Here's how the part is built. I have some questions about the finished solid (model axes, mm). A direction names the side the tool comes from. Give positions to 0.01 mm unless a question says otherwise; leave off trailing zeros. Write each loop counter-clockwise with the first axis right and the second up, starting at its lowest first coordinate (ties: lowest second). Pieces come first, ordered by that corner, then holes. Notation, with made-up numbers: (62, 6.5) - (88, 6.5) arc R18 cw to (88, 30.5) - close; hole circle Ø4 at (22.25, 8.25). An arc over 180 degrees is marked (long way). Use a Markdown table: item, result.
```python
from build123d import *

# Parameters (mm, degrees)
SKETCH1_W           = 20
SKETCH1_H           = 24
BOSS_EXTRUDE1_DEPTH = 3.5
SKETCH2_W           = 16
SKETCH2_H           = 22
CUT_EXTRUDE1_DEPTH  = 0.4
SKETCH3_R           = 1.5
CUT_EXTRUDE2_DEPTH  = 17.007810594
SKETCH4_R           = 2.5
CUT_EXTRUDE3_DEPTH  = 1
SKETCH5_R           = 1
BOSS_EXTRUDE2_DEPTH = 2


with BuildPart() as part:
    # Sketch1 → Boss-Extrude1 (new body)
    with BuildSketch(Plane.XY):
        Rectangle(SKETCH1_W, SKETCH1_H)
    extrude(amount=BOSS_EXTRUDE1_DEPTH)

    # Sketch2 → Cut-Extrude1 (cut)
    with BuildSketch(Plane(origin=(0, 0, 0), x_dir=(-1, 0, 0), z_dir=(0, 0, -1))):
        Rectangle(SKETCH2_W, SKETCH2_H)
    extrude(amount=-CUT_EXTRUDE1_DEPTH, mode=Mode.SUBTRACT)

    # Sketch3 → Cut-Extrude2 (cut, through all)
    with BuildSketch(Plane.XY.offset(3.5)):
        with Locations((0, 3)):
            Circle(SKETCH3_R)
        with Locations((0, 9)):
            Circle(SKETCH3_R)
        with Locations(Location((0, -9, 0), (0, 0, 180))):
            Circle(SKETCH3_R)
        with Locations(Location((0, -3, 0), (0, 0, 180))):
            Circle(SKETCH3_R)
    extrude(amount=-CUT_EXTRUDE2_DEPTH, mode=Mode.SUBTRACT)

    # Sketch4 → Cut-Extrude3 (cut)
    with BuildSketch(Plane.XY.offset(3.5)):
        with Locations((0, 9)):
            Circle(SKETCH4_R)
    cut_extrude3 = extrude(amount=-CUT_EXTRUDE3_DEPTH, mode=Mode.SUBTRACT)

    # Sketch-Pattern1: Cut-Extrude3 at 3 more places
    with Locations((0, -6, 0), (0, -12, 0), (0, -18, 0)):
        add(cut_extrude3, mode=Mode.SUBTRACT)

    # Sketch5 → Boss-Extrude2 (add)
    with BuildSketch(Plane.XY.offset(3.5)):
        with Locations((8, 6)):
            Circle(SKETCH5_R)
        with Locations(Location((8, -6, 0), (0, 0, 180))):
            Circle(SKETCH5_R)
    extrude(amount=BOSS_EXTRUDE2_DEPTH)


solid = part.part
```
Item 1: Will these pins go through, and if not, where does the flat tip stop? pin 1 Ø4 at (x, y) = (0, -3) entering from -Z; pin 2 Ø4 at (x, y) = (0.5, -4) entering from +Z; pin 3 Ø4 at (x, y) = (0, 3) entering from +Z.
Values:
| item | result |
|---|---|
| pin 1 | stops at z = 0.4 |
| pin 2 | stops at z = 3.5 |
| pin 3 | stops at z = 2.5 |
Item 2: Thinking about a two-plate mould opening in Y: for faces 1 (the flat face through (10, 0, 2)), 2 (the flat face through (0, -12, 2)), 3 (the cylindrical face through (0.325, -7.536, 1.465)), which applies, +Y half, -Y half, draft (parallel to the pull), parting line (faces both ways), or undercut?
Values:
| item | result |
|---|---|
| face 1 | draft |
| face 2 | -Y half |
| face 3 | undercut |
Item 3: I need wall thicknesses on line 1 along Y through (x, z) = (0, 0.9); line 2 along Y through (x, z) = (0, 3); line 3 along Z through (x, y) = (-3.75, 1.5). Which ranges of each line are inside material? Lowest first, please. Write a range as [from, to].
Values:
| item | result |
|---|---|
| line 1 | y = [-12, -10.5], [-7.5, -4.5], [-1.5, 1.5], [4.5, 7.5], [10.5, 12] |
| line 2 | y = [-12, -11.5], [-6.5, -5.5], [-0.5, 0.5], [5.5, 6.5], [11.5, 12] |
| line 3 | z = [0.4, 3.5] |
Item 4: If we section it at A-A, the plane z = 1.8: Write out the boundary of the cut face in (x, y), plus the area to 3 significant figures.
Values:
| item | result |
|---|---|
| outline | (-10, -12) - (10, -12) - (10, 12) - (-10, 12) - close; hole circle Ø3 at (0, -9); hole circle Ø3 at (0, -3); hole circle Ø3 at (0, 3); hole circle Ø3 at (0, 9) |
| area | 452 mm2 |
Item 5: If we section it at C-C, the plane x = 0: Count the separate pieces of the cut face and the enclosed holes in it, plus the area to 3 significant figures.
Values:
| item | result |
|---|---|
| separate pieces | 5 |
| enclosed holes | 0 |
| area | 30.0 mm2 |
Item 6: If we section it at D-D, the plane x = -3.75: Write out the boundary of the cut face in (y, z), plus the area to 3 significant figures.
Values:
| item | result |
|---|---|
| outline | (-12, 0) - (-11, 0) - (-11, 0.4) - (11, 0.4) - (11, 0) - (12, 0) - (12, 3.5) - (-12, 3.5) - close |
| area | 75.2 mm2 |
Item 7: For faces 4 (the flat face through (2, 3, 2.5)), 5 (the cylindrical face through (0.325, -1.536, 1.465)), 6 (the flat face through (0, 0, 0.4)), which set-ups out of +Z, -Z, +X, -X, +Y, -Y let a thin tool reach every point of the face, with its end or its side?
Values:
| item | result |
|---|---|
| face 4 | +Z |
| face 5 | +Z, -Z |
| face 6 | -Z |
Item 8: If we section it at B-B, the plane y = -9: Write out the boundary of the cut face in (x, z).
Values:
| item | result |
|---|---|
| outline | (-10, 0) - (-8, 0) - (-8, 0.4) - (-1.5, 0.4) - (-1.5, 2.5) - (-2.5, 2.5) - (-2.5, 3.5) - (-10, 3.5) - close; (1.5, 0.4) - (8, 0.4) - (8, 0) - (10, 0) - (10, 3.5) - (2.5, 3.5) - (2.5, 2.5) - (1.5, 2.5) - close |
